from build123d import *

# Parameters (mm, degrees)
SKETCH1_R               = 6
BOSS_EXTRUDE1_DEPTH     = 5
BOSS_EXTRUDE2_START     = 100
SKETCH2_R               = 6
BOSS_EXTRUDE2_DEPTH     = 100
CUT_EXTRUDE1_DEPTH      = 101.359354322
CUT_EXTRUDE1_DEPTH_BACK = 101.359354322
SKETCH3_W               = 4
SKETCH3_H               = 50
SKETCH4_R               = 6
SKETCH4_R_2             = 5
CUT_EXTRUDE2_DEPTH      = 45


with BuildPart() as part:
    # Sketch1 → Boss-Extrude1 (new body)
    with BuildSketch(Plane(origin=(0, 0, 0), x_dir=(1, 0, 0), z_dir=(0, 1, 0))):
        with Locations(Location((0, 0, 0), (0, 0, 270))):
            Circle(SKETCH1_R)
    extrude(amount=BOSS_EXTRUDE1_DEPTH)

    # Sketch2 → Boss-Extrude2 (add)
    with BuildSketch(Plane.XZ.offset(BOSS_EXTRUDE2_START)):
        with Locations(Location((0, 0, 0), (0, 0, 270))):
            Circle(SKETCH2_R)
    extrude(amount=-BOSS_EXTRUDE2_DEPTH)

    # Sketch3 → Cut-Extrude1 (cut, two sides: drawn at the far end of the back side and taken through both)
    with BuildSketch(Plane.XY.offset(-CUT_EXTRUDE1_DEPTH_BACK)):
        with Locations((0, -20)):
            Rectangle(SKETCH3_W, SKETCH3_H)
    extrude(amount=CUT_EXTRUDE1_DEPTH + CUT_EXTRUDE1_DEPTH_BACK, mode=Mode.SUBTRACT)

    # Sketch4 → Cut-Extrude2 (cut)
    with BuildSketch(Plane.XZ.offset(100)):
        with Locations(Location((0, 0, 0), (0, 0, 270))):
            Circle(SKETCH4_R)
        with Locations(Location((0, 0, 0), (0, 0, 270))):
            Circle(SKETCH4_R_2, mode=Mode.SUBTRACT)
    extrude(amount=-CUT_EXTRUDE2_DEPTH, mode=Mode.SUBTRACT)


solid = part.part
Can you work these out from the model? Positions are in its coordinate system, mm. A direction names the side the tool comes from. Give positions to 0.01 mm unless a question says otherwise; leave off trailing zeros. Loops run counter-clockwise (first coordinate to the right, second up) from the corner with the lowest first, then second, coordinate; pieces in that order, holes last. Notation, with made-up numbers: (85, 14.25) - (143, 14.25) arc R16 cw to (143, 39.25) - close; hole circle Ø6 at (-26, 50). An arc over 180 degrees is marked (long way). One line per item, written item: value.
(1) If we section it at C-C, the plane y = -11: List the corners of the cut face in (x, z) for me, plus the area to 3 significant figures.
Verdict:
outline: (-2, -5.66) - (-2, 5.66) arc R6 ccw to start; (2, -5.66) arc R6 ccw to (2, 5.66) - close
area: 66.0 mm^2
(2) I need wall thicknesses on line 1 along X through (y, z) = (-33.5, 2); line 2 along X through (y, z) = (-29, 0); line 3 along Y through (x, z) = (1.75, -2.5). Which ranges of each line are inside material? Lowest first, please.
Verdict:
line 1: -5.66 to -2, 2 to 5.66
line 2: -6 to -2, 2 to 6
line 3: -100 to -45
(3) If we section it at B-B, the plane x = 0: List the corners of the cut face in (y, z) for me.
Verdict:
outline: (-100, -5) - (-55, -5) - (-55, -6) - (-45, -6) - (-45, 6) - (-55, 6) - (-55, 5) - (-100, 5) - close
(4) If we section it at A-A, the plane z = 0: List the corners of the cut face in (x, y) for me.
Verdict:
outline: (-6, -55) - (-5, -55) - (-5, -100) - (5, -100) - (5, -55) - (6, -55) - (6, 5) - (2, 5) - (2, -45) - (-2, -45) - (-2, 5) - (-6, 5) - close
(5) If we section it at D-D, the plane y = -93: List the corners of the cut face in (x, z) for me.
Verdict:
outline: circle Ø10 at (0, 0)
(6) If we mould it in two halves opening along X, with no side actions, what happens to faces 4 (the face through (-4.88, -77.82, 1.08)), 5 (the face through (0, -45, 0)), 6 (the face through (4, 5, 0))? For each: released by +X, released by -X, zero draft, split by the parting line, or undercut.
Verdict:
face 4: split by the parting line
face 5: undercut
face 6: zero draft
(7) I'm going to push flat-ended pins straight in: pin 1 (3 mm diameter, centred on y = -9.5, z = -4.5, fed in from -X); pin 2 (5.5 mm diameter, centred on y = -21, z = -1.5, fed in from -X); pin 3 (2 mm diameter, centred on x = 0.5, z = -0.5, fed in from +Y); pin 4 (1 mm diameter, centred on y = -36, z = -3, fed in from -X). Where does each tip first touch, or does it pass through?
Verdict:
pin 1: x = -5.2
pin 2: x = -6
pin 3: y = -45
pin 4: x = -5.45
(8) On a 3-axis mill with a long thin cutter (end or side, diameter ignored), from which of +Z, -Z, +X, -X, +Y, -Y can I reach the whole of each face in a straight line? I mean faces 1 (the face through (4, -55, 4)), 2 (the face through (-4, 5, 0)), 3 (the face through (-2, -20, 0)). Say none if no direction works.
Verdict:
face 1: -Y
face 2: +Z, -Z, +X, -X, +Y
face 3: +Z, -Z, +Y
